Design review of the part built by this model. Coordinates are the model's own, in mm. Give positions to 0.01 mm unless a question says otherwise; leave off trailing zeros. Loops run counter-clockwise (first coordinate to the right, second up) from the corner with the lowest first, then second, coordinate; pieces in that order, holes last.
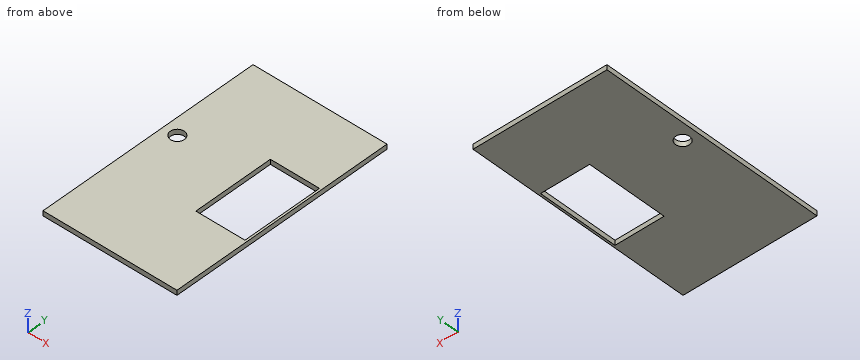
Autodesk Fusion 360 part; units mm, degrees
sketch "Sketch1" plane through (0, 0, 0) normal (0, 0, 1) x (1, 0, 0)
  line L0 (0, 0) -> (38.2, 0)
  line L1 (38.2, 0) -> (38.2, 66.3)
  line L2 (38.2, 66.3) -> (0, 66.3)
  line L3 (0, 66.3) -> (0, 0)
  dimension "d1" = 38.2
  dimension "d2" = 66.3
extrude "Extrude1" add sketch "Sketch1" along normal blind 1.3
sketch "Sketch2" plane through (0, 0, 1.3) normal (0, 0, 1) x (-1, 0, 0)
  line L0 (0, -66.3) -> (0, 0)
  line L1 (0, 0) -> (-38.2, 0)
  line L2 (-38.2, 0) -> (-38.2, -66.3)
  line L3 (-38.2, -66.3) -> (0, -66.3)
  line L4 (-0.6, -63.65) -> (-37.6, -63.65)
  line L5 (-37.6, -63.65) -> (-37.6, -2.65)
  line L6 (-37.6, -2.65) -> (-0.6, -2.65)
  line L7 (-0.6, -2.65) -> (-0.6, -63.65)
  line L8 (-37.6, -21.65) -> (-23.6, -21.65)
  line L9 (-23.6, -21.65) -> (-23.6, -44.65)
  line L10 (-23.6, -44.65) -> (-37.6, -44.65)
  line L11 (-37.6, -44.65) -> (-37.6, -21.65)
  line L12 (-0.6, -37.15) -> (-4, -37.15) construction
  circle A0 centre (-4, -37.15) radius 1.5
  dimension "d5" = 37
  dimension "d6" = 61
  dimension "d7" = 2.65
  dimension "d8" = 0.6
  dimension "d9" = 14
  dimension "d10" = 19
  dimension "d11" = 19
  dimension "d12" = 26.5
  dimension "d13" = 3
extrude "Extrude2" cut sketch "Sketch2" against normal blind 78 contours A0
extrude "Extrude3" cut sketch "Sketch2" against normal blind 2 contours L5 L8 L9 L10 L11
extrude "Extrude4" cut 1 faces at (25.4667, 66.3, 0.4333) along direction (0, -1, 0) blind 0.95
extrude "Extrude5" add 1 faces at (20.6, 7.2167, 1.3) along direction (0, 0, 1) blind 0.1
extrude "Extrude6" cut 1 faces at (25.4667, 65.35, 0.4667) along direction (0, -1, 0) blind 0.5
sketch "Sketch3" plane through (0, 0, 1.4) normal (0, 0, 1) x (-1, 0, 0)
  line L0 (-23.6, -21.65) -> (-23.6, -44.65)
  line L1 (-23.6, -44.65) -> (-37.6, -44.65)
  line L2 (-37.6, -44.65) -> (-37.6, -21.65)
  line L3 (-37.6, -21.65) -> (-23.6, -21.65)
  circle A0 centre (-4, -37.15) radius 1.5
  line L4 (-38.2, -64.85) -> (0, -64.85)
  line L5 (0, -64.85) -> (0, 0)
  line L6 (0, 0) -> (-38.2, 0)
  line L7 (-38.2, 0) -> (-38.2, -64.85)
  circle A1 centre (-4, -37.15) radius 2
  dimension "d24" = 4
extrude "Extrude7" cut sketch "Sketch3" against normal blind 4 contours A1
equation "d18 = -2.65 mm + 1.7 mm"
Q1. Take a section at A-A (x = 4). Give the boundary of the cut face in (y, z), plus the area to 3 significant figures.
Results:
outline: (0, 0) - (35.15, 0) - (35.15, 1.4) - (0, 1.4) - close; (39.15, 0) - (64.85, 0) - (64.85, 1.4) - (39.15, 1.4) - close
area: 85.2 mm2
Q2. Take a section at D-D (x = 25.5). Give the boundary of the cut face in (y, z).
Results:
outline: (0, 0) - (21.65, 0) - (21.65, 1.4) - (0, 1.4) - close; (44.65, 0) - (64.85, 0) - (64.85, 1.4) - (44.65, 1.4) - close
Q3. Take a section at B-B (y = 37.15). Give the boundary of the cut face in (x, z).
Results:
outline: (0, 0) - (2, 0) - (2, 1.4) - (0, 1.4) - close; (6, 0) - (23.6, 0) - (23.6, 1.4) - (6, 1.4) - close; (37.6, 0) - (38.2, 0) - (38.2, 1.4) - (37.6, 1.4) - close
Q4. Wall thickness on line 1 (X direction, y = 37.15, z = 0.55); line 2 (Y direction, x = 27.5, z = 1.25); line 3 (X direction, y = 24, z = 0.9): over which ranges is each line inside the solid? List them lowest first.
Results:
line 1: x = 0 to 2, 6 to 23.6, 37.6 to 38.2
line 2: y = 0 to 21.65, 44.65 to 64.85
line 3: x = 0 to 23.6, 37.6 to 38.2
Q5. Insertion check: pin 1 (0.7 mm diameter, centred on y = 35, z = 1, fed in from -X); pin 2 (3 mm diameter, centred on x = 4, y = 37.15, fed in from -Z). Each pin has a flat end and moves straight along its axis. Give the tip position at first contact, or say it passes through.
Results:
pin 1: stops at x = 0
pin 2: passes through
Q6. Take a section at C-C (z = 0.45). Give the boundary of the cut face in (x, y), plus the area to 3 significant figures.
Results:
outline: (0, 0) - (38.2, 0) - (38.2, 64.85) - (0, 64.85) - close; hole circle Ø4 at (4, 37.15); hole (23.6, 21.65) - (37.6, 21.65) - (37.6, 44.65) - (23.6, 44.65) - close
area: 2,140 mm2
